from build123d import *

# Parameters (mm, degrees)
SKETCH1_W              = 140
SKETCH1_H              = 152
BOSS_EXTRUDE1_DEPTH    = 5
SKETCH2_R              = 3.05
SKETCH2_R_2            = 8
SKETCH2_R_3            = 6.5
CUT_EXTRUDE1_DEPTH     = 104.445637897
SKETCH4_W              = 8
SKETCH4_H              = 36
CUT_EXTRUDE3_DEPTH     = 104.445637897
CUT_EXTRUDE2_DEPTH     = 104.445637897
FILLET3_R              = 1.5
LPATTERN1_COUNT        = 3
LPATTERN1_PITCH        = 50
FILLET3_OF_LPATTERN1_R = 1.5
LPATTERN4_DEPTH        = 5
FILLET1_R              = 4


# Read off the part's stored shape, not the designer's step: LPattern4
with BuildPart() as part:
    # Sketch1 → Boss-Extrude1 (new body)
    with BuildSketch(Plane(origin=(0, 0, 0), x_dir=(1, 0, 0), z_dir=(0, 1, 0))):
        Rectangle(SKETCH1_W, SKETCH1_H)
    extrude(amount=BOSS_EXTRUDE1_DEPTH)

    # Sketch2 → Cut-Extrude1 (cut, through all)
    with BuildSketch(Plane(origin=(0, 5, 0), x_dir=(1, 0, 0), z_dir=(0, 1, 0))):
        with Locations(Location((-50, 0, 0), (0, 0, 270))):
            Circle(SKETCH2_R)
        with Locations(Location((-25, 0, 0), (0, 0, 270))):
            Circle(SKETCH2_R_2)
        with Locations(Location((-40, -10, 0), (0, 0, 270))):
            Circle(SKETCH2_R_3)
    cut_extrude1 = extrude(amount=-CUT_EXTRUDE1_DEPTH, mode=Mode.SUBTRACT)

    # Mirror1: Cut-Extrude1 across plane
    add(cut_extrude1.mirror(Plane(origin=(0, 0, 0), x_dir=(0, 0, 1), z_dir=(1, 0, 0))), mode=Mode.SUBTRACT)

    # Sketch4 → Cut-Extrude3 (cut, through all)
    with BuildSketch(Plane(origin=(0, 5, 0), x_dir=(1, 0, 0), z_dir=(0, 1, 0))):
        with Locations((-66, 0)):
            Rectangle(SKETCH4_W, SKETCH4_H)
    extrude(amount=-CUT_EXTRUDE3_DEPTH, mode=Mode.SUBTRACT)

    # Sketch3 → Cut-Extrude2 (cut, through all)
    with BuildSketch(Plane(origin=(0, 5, 0), x_dir=(1, 0, 0), z_dir=(0, 1, 0))):
        with BuildLine():
            ThreePointArc((-42, -26), (-42.878679656, -28.121320344), (-45, -29))
            Line((-45, -29), (-46.5, -29))
            Line((-46.5, -29), (-46.5, -38.5))
            Line((-46.5, -38.5), (-33, -38.5))
            Line((-33, -38.5), (-33, -22))
            Line((-33, -22), (-42, -22))
            Line((-42, -22), (-42, -26))
        make_face()
    cut_extrude2 = extrude(amount=-CUT_EXTRUDE2_DEPTH, mode=Mode.SUBTRACT)

    # Fillet3
    fillet3_edges = [part.edges().sort_by_distance(p)[0] for p in [
        (-33, 2.5, 38.5),
        (-46.5, 2.5, 38.5),
        (-46.5, 2.5, 29),
        (-33, 2.5, 22),
        (-42, 2.5, 22),
    ]]
    fillet(fillet3_edges, radius=FILLET3_R - 0.0001)  # a hair under: the kernel refuses the full size

    # LPattern1: Cut-Extrude2 ×3
    with Locations(*[(i * LPATTERN1_PITCH, 0, 0) for i in range(1, LPATTERN1_COUNT)]):
        add(cut_extrude2, mode=Mode.SUBTRACT)

    # Fillet3 of LPattern1
    fillet3_of_lpattern1_edges = [part.edges().sort_by_distance(p)[0] for p in [
        (17, 2.5, 38.5),
        (3.5, 2.5, 38.5),
        (3.5, 2.5, 29),
        (17, 2.5, 22),
        (8, 2.5, 22),
        (67, 2.5, 38.5),
        (53.5, 2.5, 38.5),
        (53.5, 2.5, 29),
        (67, 2.5, 22),
        (58, 2.5, 22),
    ]]
    fillet(fillet3_of_lpattern1_edges, radius=FILLET3_OF_LPATTERN1_R - 0.0001)  # a hair under: the kernel refuses the full size

    # LPattern4 outline → LPattern4 (cut)
    with BuildSketch(Plane(origin=(0, 0, 0), x_dir=(1, 0, 0), z_dir=(0, 1, 0))):
        with BuildLine():
            ThreePointArc((65.5, 56.5), (66.560660172, 56.939339828), (67, 58))
            Line((67, 58), (67, 71.5))
            ThreePointArc((67, 71.5), (66.560660172, 72.560660172), (65.5, 73))
            Line((65.5, 73), (59.5, 73))
            ThreePointArc((59.5, 73), (58.439339828, 72.560660172), (58, 71.5))
            Line((58, 71.5), (58, 69))
            ThreePointArc((58, 69), (57.121320344, 66.878679656), (55, 66))
            ThreePointArc((55, 66), (53.939339828, 65.560660172), (53.5, 64.5))
            Line((53.5, 64.5), (53.5, 58))
            ThreePointArc((53.5, 58), (53.939339828, 56.939339828), (55, 56.5))
            Line((55, 56.5), (65.5, 56.5))
        make_face()
        with BuildLine():
            Line((-42, 71.5), (-42, 69))
            ThreePointArc((-42, 69), (-42.878679656, 66.878679656), (-45, 66))
            ThreePointArc((-45, 66), (-46.060660172, 65.560660172), (-46.5, 64.5))
            Line((-46.5, 64.5), (-46.5, 58))
            ThreePointArc((-46.5, 58), (-46.060660172, 56.939339828), (-45, 56.5))
            Line((-45, 56.5), (-34.5, 56.5))
            ThreePointArc((-34.5, 56.5), (-33.439339828, 56.939339828), (-33, 58))
            Line((-33, 58), (-33, 71.5))
            ThreePointArc((-33, 71.5), (-33.439339828, 72.560660172), (-34.5, 73))
            Line((-34.5, 73), (-40.5, 73))
            ThreePointArc((-40.5, 73), (-41.560660172, 72.560660172), (-42, 71.5))
        make_face()
        with BuildLine():
            Line((8, 71.5), (8, 69))
            ThreePointArc((8, 69), (7.121320344, 66.878679656), (5, 66))
            ThreePointArc((5, 66), (3.939339828, 65.560660172), (3.5, 64.5))
            Line((3.5, 64.5), (3.5, 58))
            ThreePointArc((3.5, 58), (3.939339828, 56.939339828), (5, 56.5))
            Line((5, 56.5), (15.5, 56.5))
            ThreePointArc((15.5, 56.5), (16.560660172, 56.939339828), (17, 58))
            Line((17, 58), (17, 71.5))
            ThreePointArc((17, 71.5), (16.560660172, 72.560660172), (15.5, 73))
            Line((15.5, 73), (9.5, 73))
            ThreePointArc((9.5, 73), (8.439339828, 72.560660172), (8, 71.5))
        make_face()
    extrude(amount=LPATTERN4_DEPTH, mode=Mode.SUBTRACT)

    # Fillet1
    fillet1_edges = [part.edges().sort_by_distance(p)[0] for p in [
        (-70, 2.5, -76),
        (70, 2.5, -76),
        (70, 2.5, 76),
        (-70, 2.5, 76),
        (-70, 2.5, 18),
        (-62, 2.5, 18),
        (-62, 2.5, -18),
        (-70, 2.5, -18),
    ]]
    fillet(fillet1_edges, radius=FILLET1_R - 0.0001)  # a hair under: the kernel refuses the full size


solid = part.part
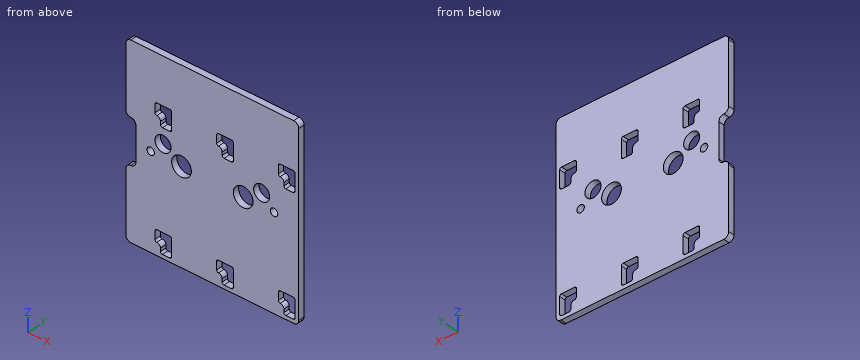
Verification items for the finished model (mm, model axes). Round coordinates to 2 decimals unless told otherwise and drop trailing zeros. Write each loop counter-clockwise with the first axis right and the second up, starting at its lowest first coordinate (ties: lowest second). Pieces come first, ordered by that corner, then holes.
(1) Material ranges on line 1 (X direction, y = 1.75, z = 0); line 2 (X direction, y = 2.55, z = 10); line 3 (Z direction, x = 61, y = 3.15), recorded low to high.
Returned:
line 1: x = -62 to -53.05, -46.95 to -33, -17 to 17, 33 to 46.95, 53.05 to 70
line 2: x = -62 to -46.5, -33.5 to 33.5, 46.5 to 70
line 3: z = -76 to -73, -56.5 to 22, 38.5 to 76
(2) Section check D-D (y = 1.5). Give the number of separate pieces and of enclosed holes in the cut face, plus the area to 3 significant figures.
Returned:
separate pieces: 1
enclosed holes: 12
area: 19,100 mm2
(3) Section check A-A (x = 11.5). Enter the section's corners in (y, z).
Returned:
outline: (0, -76) - (5, -76) - (5, -73) - (0, -73) - close; (0, -56.5) - (5, -56.5) - (5, 22) - (0, 22) - close; (0, 38.5) - (5, 38.5) - (5, 76) - (0, 76) - close
(4) Section check C-C (x = 50). Enter the section's corners in (y, z), plus the area to 4 significant figures.
Returned:
outline: (0, -76) - (5, -76) - (5, -3.05) - (0, -3.05) - close; (0, 3.05) - (5, 3.05) - (5, 76) - (0, 76) - close
area: 729.5 mm2
(5) Section check B-B (z = 0). Enter the section's corners in (x, y).
Returned:
outline: (-62, 0) - (-53.05, 0) - (-53.05, 5) - (-62, 5) - close; (-46.95, 0) - (-33, 0) - (-33, 5) - (-46.95, 5) - close; (-17, 0) - (17, 0) - (17, 5) - (-17, 5) - close; (33, 0) - (46.95, 0) - (46.95, 5) - (33, 5) - close; (53.05, 0) - (70, 0) - (70, 5) - (53.05, 5) - close
